For this review, take the finished solid that the model builds, in its own axes (mm). A direction names the side the tool comes from. Give positions to 0.01 mm unless a question says otherwise; leave off trailing zeros. Loops run counter-clockwise (first coordinate to the right, second up) from the corner with the lowest first, then second, coordinate; pieces in that order, holes last. Notation, with made-up numbers: (-22, -24.5) - (-7, -24.5) arc R20 ccw to (-7, 13.5) - close; hole circle Ø6 at (36.5, 57.25). An arc over 180 degrees is marked (long way). Use CSV: the item, a comma, the result in double quotes. Start each with the question number.
1. Take a section at B-B on y = 11.5. State how many separate pieces and enclosed holes the cut face has, plus the area to 3 significant figures.
2. Wall thickness on line 1 (Y direction, x = 0, z = 3); line 2 (X direction, y = 0, z = 2.8); line 3 (X direction, y = 5, z = 2.5): over which ranges is each line inside the solid? List them lowest first.
3. Take a section at A-A on z = 2.5. Give the boundary of the cut face in (x, y), plus the area to 3 significant figures.
4. For faces 4 (the flat face through (60.25, 7, 3)), 5 (the flat face through (60, 4.5, 2)), 6 (the flat face through (66, 9, -3.5)), 7 (the flat face through (64, 12.5, 9)), list the 3-axis set-ups (+Z, -Z, +X, -X, +Y, -Y) from which the entire face can be reached by the end or side of a thin tool; tool diameter is ignored.
5. Mouldability with a two-part tool opening along X and no side actions: class faces 1 (the flat face through (17.4, -0.1, 0)), 2 (the flat face through (55, 1, 2)), 3 (the flat face through (52.75, 11, 3)) as pulls with the +X half, pulls with the -X half, needs draft (parallel to the pull), parting line crosses it, or undercut.
6. For pin 1 (5.5 mm diameter, centred on x = 44.5, z = 2.5, fed in from -Y); pin 2 (1 mm diameter, centred on x = 79.5, y = 8, fed in from -Z); pin 3 (6.5 mm diameter, centred on y = 7, z = -0.5, fed in from -X); pin 4 (3 mm diameter, centred on x = 62.5, y = 2, fed in from -Z) (1 decimal), all flat-tipped, find the tip position at first contact; note any pin that passes through.
```python
from build123d import *
from build123d.topology import SkipClean

# Parameters (mm, degrees)
BOSS_EXTRUDE1_DEPTH = 5
CHAMFER2_SIZE       = 1.5
CHAMFER2_SIZE2      = 0.699461487
FILLET1_R           = 10
SKETCH10_W          = 32
SKETCH10_H          = 5
BOSS_EXTRUDE3_DEPTH = 2
SKETCH5_W           = 32
SKETCH5_H           = 16
BOSS_EXTRUDE2_DEPTH = 8
SKETCH6_W           = 22.5
SKETCH6_H           = 12
CUT_EXTRUDE1_DEPTH  = 4
SKETCH7_W           = 25
SKETCH7_H           = 5
CUT_EXTRUDE2_DEPTH  = 7
SKETCH8_W           = 15
SKETCH8_H           = 12
CUT_EXTRUDE3_DEPTH  = 86.571607441
CUT_EXTRUDE4_DEPTH  = 85.32378075
FILLET2_R           = 2
FILLET3_START       = 48
FILLET3_DEPTH       = 6.9999999
FILLET3_START_2     = 47.322875556
FILLET3_2_DEPTH     = 9.677124544
FILLET3_START_3     = -3
FILLET3_3_DEPTH     = 10
FILLET4_R           = 3


with BuildPart() as part:
    # Sketch1 → Boss-Extrude1 (new body)
    with BuildSketch(Plane.XY):
        with BuildLine():
            ThreePointArc((16.815171721, -2.5), (-17, 0), (16.815171721, 2.5))
            Line((16.815171721, 2.5), (19.843134833, 2.5))
            ThreePointArc((19.843134833, 2.5), (-20, 0), (19.843134833, -2.5))
            Line((19.843134833, -2.5), (16.815171721, -2.5))
        make_face()
        with BuildLine():
            Line((19.843134833, 2.5), (16.815171721, 2.5))
            ThreePointArc((16.815171721, 2.5), (16.953729962, 1.253411494), (17, 0))
            ThreePointArc((17, 0), (16.953729962, -1.253411494), (16.815171721, -2.5))
            Line((16.815171721, -2.5), (19.843134833, -2.5))
            ThreePointArc((19.843134833, -2.5), (19.960745185, -1.252458251), (20, 0))
            ThreePointArc((20, 0), (19.960745185, 1.252458251), (19.843134833, 2.5))
        make_face()
        with BuildLine():
            Line((80, 2.5), (19.843134833, 2.5))
            ThreePointArc((19.843134833, 2.5), (19.960745185, 1.252458251), (20, 0))
            ThreePointArc((20, 0), (19.960745185, -1.252458251), (19.843134833, -2.5))
            Line((19.843134833, -2.5), (80, -2.5))
            Line((80, -2.5), (80, 2.5))
        make_face()
    extrude(amount=BOSS_EXTRUDE1_DEPTH)

    # Chamfer2
    chamfer2_edges = [part.edges().sort_by_distance(p)[0] for p in [
        (-16.815171721, -2.5, 5),
    ]]
    chamfer2_side = [part.faces().sort_by_distance(p)[0] for p in [
        (23.12129627, 0, 5),
    ]]
    chamfer(chamfer2_edges, length=CHAMFER2_SIZE, length2=CHAMFER2_SIZE2, reference=chamfer2_side[0])

    # Fillet1
    fillet1_edges = [part.edges().sort_by_distance(p)[0] for p in [
        (19.843134833, 2.5, 2.5),
        (19.843134833, -2.5, 2.5),
    ]]
    fillet(fillet1_edges, radius=FILLET1_R)

    # Sketch10 → Boss-Extrude3 (add)
    with BuildSketch(Plane(origin=(0, 2.5, 0), x_dir=(1, 0, 0), z_dir=(0, 1, 0))):
        with Locations((64, -2.5)):
            Rectangle(SKETCH10_W, SKETCH10_H)
    extrude(amount=BOSS_EXTRUDE3_DEPTH)

    # Sketch5 → Boss-Extrude2 (add)
    with BuildSketch(Plane(origin=(0, 4.5, 0), x_dir=(1, 0, 0), z_dir=(0, 1, 0))):
        with Locations((64, -2.5)):
            Rectangle(SKETCH5_W, SKETCH5_H)
    extrude(amount=BOSS_EXTRUDE2_DEPTH)

    # Sketch6 → Cut-Extrude1 (cut)
    with BuildSketch(Plane(origin=(0, 12.5, 0), x_dir=(1, 0, 0), z_dir=(0, 1, 0))):
        with Locations((64, -2.5)):
            Rectangle(SKETCH6_W, SKETCH6_H)
    extrude(amount=-CUT_EXTRUDE1_DEPTH, mode=Mode.SUBTRACT)

    # Sketch7 → Cut-Extrude2 (cut)
    with BuildSketch(Plane.XZ.offset(2.5)):
        with Locations((67.5, 2.5)):
            Rectangle(SKETCH7_W, SKETCH7_H)
    extrude(amount=-CUT_EXTRUDE2_DEPTH, mode=Mode.SUBTRACT)

    # Sketch8 → Cut-Extrude3 (cut, through all)
    with BuildSketch(Plane(origin=(0, 8.5, 0), x_dir=(1, 0, 0), z_dir=(0, 1, 0))):
        with Locations((67.75, -2.5)):
            Rectangle(SKETCH8_W, SKETCH8_H)
    extrude(amount=-CUT_EXTRUDE3_DEPTH, mode=Mode.SUBTRACT)

    # Sketch9 → Cut-Extrude4 (cut, through all)
    with BuildSketch(Plane.XZ.offset(-4.5)):
        with BuildLine():
            Line((78, 4), (80, 4))
            Line((80, 4), (80, 1))
            Line((80, 1), (78, 1))
            ThreePointArc((78, 1), (76.5, 2.5), (78, 4))
        make_face()
    extrude(amount=-CUT_EXTRUDE4_DEPTH, mode=Mode.SUBTRACT)

    # Fillet2
    fillet2_edges = [part.edges().sort_by_distance(p)[0] for p in [
        (55, 4.5, 2.5),
        (48, 2.5, 2.5),
        (55, -2.5, 2.5),
    ]]
    fillet(fillet2_edges, radius=FILLET2_R)

    # Fillet3: read off the stored shape, not the designer's step
    # Fillet3 outline → Fillet3 (add)
    with BuildSketch(Plane.YZ.offset(FILLET3_START)):
        with BuildLine():
            Line((4.5, -1.5), (4.5, 0))
            Line((4.5, 0), (3, 0))
            ThreePointArc((3, 0), (4.060660172, -0.439339828), (4.5, -1.5))
        make_face()
        with BuildLine():
            ThreePointArc((4.5, 6.5), (4.060660172, 5.439339828), (3, 5))
            Line((3, 5), (4.5, 5))
            Line((4.5, 5), (4.5, 6.5))
        make_face()
    extrude(amount=FILLET3_DEPTH)

    # Fillet3 2 outline → Fillet3 2 (add)
    with BuildSketch(Plane.YZ.offset(FILLET3_START_2)):
        with BuildLine():
            Line((4.5, -1.5), (4.5, 0))
            Line((4.5, 0), (3, 0))
            ThreePointArc((3, 0), (4.060660172, -0.439339828), (4.5, -1.5))
        make_face()
        with BuildLine():
            ThreePointArc((4.5, 6.5), (4.060660172, 5.439339828), (3, 5))
            Line((3, 5), (4.5, 5))
            Line((4.5, 5), (4.5, 6.5))
        make_face()
    extrude(amount=FILLET3_2_DEPTH)

    # Fillet3 3 outline → Fillet3 3 (cut)
    with SkipClean():  # the faces are left unmerged after this step: merging them gives an invalid solid
        with BuildSketch(Plane.XY.offset(FILLET3_START_3)):
            with BuildLine():
                Line((47.322875556, 4.5), (47.3228756, 2.999999951))
                ThreePointArc((47.3228756, 2.999999951), (47.82287564, 3.67712431), (48, 4.5))
                Line((48, 4.5), (47.322875556, 4.5))
            make_face()
            with BuildLine():
                ThreePointArc((57, 4.5), (55.775255129, 4.08113883), (55.063508327, 3))
                Line((55.063508327, 3), (57.0000001, 3))
                Line((57.0000001, 3), (57, 4.5))
            make_face()
        extrude(amount=FILLET3_3_DEPTH, mode=Mode.SUBTRACT)
    add(part.part.scale(1), mode=Mode.REPLACE)  # the faces are merged on a copy

    # Fillet4
    fillet4_edges = [part.edges().sort_by_distance(p)[0] for p in [
        (80, 8.5, 10.5),
        (80, 8.5, -5.5),
        (48, 8.5, -5.5),
        (48, 8.5, 10.5),
    ]]
    fillet(fillet4_edges, radius=FILLET4_R)


solid = part.part
```
Check result:
1,separate pieces,"3"
1,enclosed holes,"1"
1,area,"262 mm²"
2,line 1,"y = -20 to -17, 17 to 20"
2,line 2,"x = -20 to -17, 17 to 55"
2,line 3,"x = -19.36 to -16.25, 16.25 to 20.66, 48 to 60.25, 75.25 to 76.5"
3,outline,"(18.18, -8.33) arc R10 cw to (27.27, -2.5) - (53, -2.5) arc R2 ccw to (55, -0.5) - (55, 2.5) arc R2 cw to (57, 4.5) - (60.25, 4.5) - (60.25, 8.5) - (52.75, 8.5) - (52.75, 12.5) - (48, 12.5) - (48, 4.5) arc R2 cw to (46, 2.5) - (27.27, 2.5) arc R10 cw to (18.18, 8.33) arc R20 ccw (long way) to start; (75.25, 4.5) - (76.5, 4.5) - (76.5, 12.5) - (75.25, 12.5) - close; hole circle Ø34 at (0, 0)"
3,area,"635 mm²"
4,face 4,"+Y, -Y"
4,face 5,"+X, -Y"
4,face 6,"+Y"
4,face 7,"+Z, -Z, +X, +Y"
5,face 1,"needs draft"
5,face 2,"pulls with the +X half"
5,face 3,"undercut"
6,pin 1,"stops at y = -2.5"
6,pin 2,"stops at z = -4.74"
6,pin 3,"stops at x = -19.64"
6,pin 4,"passes through"
